CAD build for the part. Positions are in the model's coordinates, mm. A direction names the side the tool comes from. Give positions to 0.01 mm unless a question says otherwise; leave off trailing zeros. Loops run counter-clockwise (first coordinate to the right, second up) from the corner with the lowest first, then second, coordinate; pieces in that order, holes last. Notation, with made-up numbers: (-7, 0) - (24, 0) arc R13 cw to (24, 7) - close; hole circle Ø3 at (88, 35.25). An arc over 180 degrees is marked (long way). Return JSON: item names as keys, results as strings.
from build123d import *

# Parameters (mm, degrees)
SKETCH1_R           = 37.5
BOSS_EXTRUDE1_DEPTH = 72
CUT_EXTRUDE1_START  = -25
SKETCH3_R           = 37.5
SKETCH3_R_2         = 37
CUT_EXTRUDE1_DEPTH  = 25
CUT_EXTRUDE2_START  = -25
SKETCH2_R           = 37.5
SKETCH2_R_2         = 37
CUT_EXTRUDE2_DEPTH  = 25
SKETCH5_R           = 5
CUT_EXTRUDE3_DEPTH  = 70
SKETCH6_W           = 10
SKETCH6_H           = 40
CUT_EXTRUDE4_DEPTH  = 5


with BuildPart() as part:
    # Sketch1 → Boss-Extrude1 (new body)
    with BuildSketch(Plane(origin=(0, 0, 0), x_dir=(1, 0, 0), z_dir=(0, 1, 0))):
        with Locations(Location((0, 0, 0), (0, 0, 270))):
            Circle(SKETCH1_R)
    extrude(amount=BOSS_EXTRUDE1_DEPTH)

    # Sketch3 → Cut-Extrude1 (cut)
    with BuildSketch(Plane(origin=(0, 65, 0), x_dir=(1, 0, 0), z_dir=(0, 1, 0)).offset(CUT_EXTRUDE1_START)):
        with Locations(Location((0, 0, 0), (0, 0, 270))):
            Circle(SKETCH3_R)
        with Locations(Location((0, 0, 0), (0, 0, 270))):
            Circle(SKETCH3_R_2, mode=Mode.SUBTRACT)
    extrude(amount=CUT_EXTRUDE1_DEPTH, mode=Mode.SUBTRACT)

    # Sketch2 → Cut-Extrude2 (cut)
    with BuildSketch(Plane(origin=(0, 26, 0), x_dir=(1, 0, 0), z_dir=(0, 1, 0)).offset(CUT_EXTRUDE2_START)):
        with Locations(Location((0, 0, 0), (0, 0, 270))):
            Circle(SKETCH2_R)
        with Locations(Location((0, 0, 0), (0, 0, 270))):
            Circle(SKETCH2_R_2, mode=Mode.SUBTRACT)
    extrude(amount=CUT_EXTRUDE2_DEPTH, mode=Mode.SUBTRACT)

    # Loft2: read off the stored shape, not the designer's step
    # Loft2: loft between two sections, ruled curve by curve
    loft2_from = [
        Edge.make_bspline([(-14.77077476, -10, 20.169883812), (25.568992863, -10, 49.711433333), (55.110542384, -10, 9.371665709), (14.77077476, -10, -20.169883812), (-25.568992863, -10, -49.711433333), (-55.110542384, -10, -9.371665709), (-14.77077476, -10, 20.169883812)], [0, 0, 0, 0, 0.5, 0.5, 0.5, 1, 1, 1, 1], 3, [1, 0.333333333, 0.333333333, 1, 0.333333333, 0.333333333, 1]),
    ]
    loft2_to = [
        Edge.make_bspline([(-12.502949146, 0, 35.354296241), (58.205643335, 0, 60.360194532), (83.211541627, 0, -10.348397949), (12.502949146, 0, -35.354296241), (-58.205643335, 0, -60.360194532), (-83.211541627, 0, 10.348397949), (-12.502949146, 0, 35.354296241)], [0, 0, 0, 0, 0.5, 0.5, 0.5, 1, 1, 1, 1], 3, [1, 0.333333333, 0.333333333, 1, 0.333333333, 0.333333333, 1]),
    ]
    loft2 = Solid(Shell([*[Face.make_surface_from_curves(loft2_from[k], loft2_to[k]) for k in range(1)], Face(Wire(loft2_from)), Face(Wire(loft2_to))]))
    add(loft2)

    # Sketch5 → Cut-Extrude3 (cut)
    with BuildSketch(Plane(origin=(0, 72, 0), x_dir=(1, 0, 0), z_dir=(0, 1, 0))):
        with Locations(Location((0, 0, 0), (0, 0, 270))):
            Circle(SKETCH5_R)
    extrude(amount=-CUT_EXTRUDE3_DEPTH, mode=Mode.SUBTRACT)

    # Sketch6 → Cut-Extrude4 (cut)
    with BuildSketch(Plane.XZ.offset(10)):
        Rectangle(SKETCH6_W, SKETCH6_H)
    extrude(amount=-CUT_EXTRUDE4_DEPTH, mode=Mode.SUBTRACT)


solid = part.part
1. Cut at B-B, the plane y = 13. Write the cut outline in (x, z).
Values follow:
{"outline": "circle Ø74 at (0, 0); hole circle Ø10 at (0, 0)"}
2. Drill centre lines: probe 1 along X at (y, z) = (29, 0); probe 2 along X at (y, z) = (25.5, 0); probe 3 along X at (y, z) = (-3, 20.5). Where is each one in solid material? Low to high.
Values follow:
{"probe 1": "x = -37.5 to -5, 5 to 37.5", "probe 2": "x = -37 to -5, 5 to 37", "probe 3": "x = -26.5 to 26.5"}
3. Drop flat-ended pins along their axis: P1, Ø3, axis at x = -2, z = 5.5, coming from the -Y side; P2, Ø6, axis at y = 35.5, z = -3, coming from the +X side; P3, Ø1.5, axis at y = 33.5, z = 15.5, coming from the +X side. Give the stop position or say it passes through.
Values follow:
{"P1": "stops at y = -5", "P2": "stops at x = 37.5", "P3": "stops at x = 34.48"}
4. Pull direction Y, two halves, no side cores. Call faces 4 (the face through (0, -5, 0)), 5 (the face through (-33.2, 40, -16.8)), 6 (the face through (-8, 72, -1)): +Y half, -Y half, draft (parallel to the pull), parting line (faces both ways), or undercut.
Values follow:
{"face 4": "-Y half", "face 5": "undercut", "face 6": "+Y half"}
5. Cut at A-A, the plane y = 30. Write the cut outline in (x, z), plus the area to 3 significant figures.
Values follow:
{"outline": "circle Ø75 at (0, 0); hole circle Ø10 at (0, 0)", "area": "4,340 mm²"}
6. Which spindle directions (+Z, -Z, +X, -X, +Y, -Y) get a long thin tool onto all of the face, cutting with end or side? Do faces 1 (the face through (0, -8, -20)), 2 (the face through (-14.17, 52.32, 34.18)), 3 (the face through (-4.88, 37.49, -1.08)). Say none if no direction does.
Values follow:
{"face 1": "-Y", "face 2": "none", "face 3": "+Y"}
